from build123d import *

# Parameters (mm, degrees)
SKETCH_2_W                       = 40
SKETCH_2_H                       = 17
SM_BASE_FLANGE_1_DEPTH           = 2
SM_EDGE_FLANGE_1_STRIP_W         = 9.4732
SM_EDGE_FLANGE_1_STRIP_H         = 2
SM_EDGE_FLANGE_1_STRIP_CUT_DEPTH = 40
SM_EDGE_FLANGE_1_DEPTH           = 40
SKETCH_10_R                      = 3.3
CUT_EXTRUDE_1_DEPTH              = 10
FILLET_1_R                       = 6
FILLET_2_R                       = 2


# Sheet-metal steps are written as plain solids
with BuildPart() as part:
    # Sketch 2 → 基体-法兰1 (new body)
    with BuildSketch(Plane.XY):
        Rectangle(SKETCH_2_W, SKETCH_2_H)
    extrude(amount=-SM_BASE_FLANGE_1_DEPTH)

    # 边线-法兰1 strip (across the edge) → 边线-法兰1 strip cut (cut)
    with BuildSketch(Plane(origin=(-20, 8.5, -2), x_dir=(0, -1, 0), z_dir=(1, 0, 0))):
        with Locations((-2, -1)):
            Rectangle(SM_EDGE_FLANGE_1_STRIP_W, SM_EDGE_FLANGE_1_STRIP_H)
    extrude(amount=SM_EDGE_FLANGE_1_STRIP_CUT_DEPTH, mode=Mode.SUBTRACT)

    # 边线-法兰1 section (across the edge) → 边线-法兰1 (add)
    with BuildSketch(Plane(origin=(-20, 8.5, -2), x_dir=(0, -1, 0), z_dir=(1, 0, 0))):
        with BuildLine():
            Line((0, 0.7366), (0, 13))
            Line((0, 13), (2, 13))
            Line((2, 13), (2, 0.7366))
            ThreePointArc((2, 0.7366), (2.215745145, 0.215745145), (2.7366, 0))
            Line((2.7366, 0), (2.7366, -2))
            ThreePointArc((2.7366, -2), (0.801531583, -1.198468417), (0, 0.7366))
        make_face()
    extrude(amount=SM_EDGE_FLANGE_1_DEPTH)

    # 草图10 → 切除-拉伸1 (cut)
    with BuildSketch(Plane(origin=(0, 0, -2), x_dir=(-1, 0, 0), z_dir=(0, 0, -1))):
        with Locations((-12.5, -2.5)):
            Circle(SKETCH_10_R)
        with Locations((12.5, -2.5)):
            Circle(SKETCH_10_R)
    extrude(amount=-CUT_EXTRUDE_1_DEPTH, mode=Mode.SUBTRACT)

    # 圆角1
    fillet_1_edges = [part.edges().sort_by_distance(p)[0] for p in [
        (20, -8.5, -1),
        (-20, -8.5, -1),
    ]]
    fillet(fillet_1_edges, radius=FILLET_1_R)

    # 圆角2
    fillet_2_edges = [part.edges().sort_by_distance(p)[0] for p in [
        (-20, 7.5, -15),
        (20, 7.5, -15),
    ]]
    fillet(fillet_2_edges, radius=FILLET_2_R)


solid = part.part
CAD build for the part. Positions are in the model's coordinates, mm. A direction names the side the tool comes from. Coordinates: 2 decimals unless noted, no trailing zeros. Loops run counter-clockwise (first coordinate to the right, second up) from the corner with the lowest first, then second, coordinate; pieces in that order, holes last. Notation, with made-up numbers: (-2, 59.5) -> (25, 59.5) arc R22 cw to (25, 68.5) -> close; hole circle Ø9 at (4, 78.25). An arc over 180 degrees is marked (long way). One line per item, written item: value.
1. Flat gauge pin, fed straight in: P1, Ø7, axis at x = -3, y = 1.5, coming from the -Z side. Where does the tip first touch, or does it go through?
Answers:
P1: stops at z = -2
2. Slice it at D-D on y = 7.75. Write the cut outline in (x, z).
Answers:
outline: (-20, -13) arc R2 ccw to (-18, -15) -> (18, -15) arc R2 ccw to (20, -13) -> (20, -0.85) -> (-20, -0.85) -> close
3. Drill centre lines: line 1 (Y direction, x = -4.5, z = -12); line 2 (Z direction, x = 16, y = 4.25); line 3 (Y direction, x = -12.5, z = -1). Where is each one in solid material? Low to high. Write a range as [from, to].
Answers:
line 1: y = [6.5, 8.5]
line 2: z = [-2, 0]
line 3: y = [-8.5, -5.8], [0.8, 7.88]
4. Pull direction Y, two halves, no side cores. Call faces 1 (the face through (0, 8.5, -9)), 2 (the face through (-19.43, 7.49, -14.4)), 3 (the face through (-9.2, -2.4, -1)), 4 (the face through (18.289, -6.696, -1.014)): pulls with the +Y half, pulls with the -Y half, needs draft (parallel to the pull), parting line crosses it, or undercut.
Answers:
face 1: pulls with the +Y half
face 2: needs draft
face 3: undercut
face 4: pulls with the -Y half
5. Which spindle directions (+Z, -Z, +X, -X, +Y, -Y) get a long thin tool onto all of the face, cutting with end or side? Do faces 5 (the face through (0, 6.5, -9)), 6 (the face through (0, 8, -15)). Say none if no direction does.
Answers:
face 5: -Z, +X, -X, -Y
face 6: -Z, +X, -X, +Y, -Y
6. Slice it at B-B on z = -1.25. Write the cut outline in (x, y), and give its area (3 significant figures).
Answers:
outline: (-20, -2.5) arc R6 ccw to (-14, -8.5) -> (14, -8.5) arc R6 ccw to (20, -2.5) -> (20, 8.06) -> (-20, 8.06) -> close; hole circle Ø6.6 at (-12.5, -2.5); hole circle Ø6.6 at (12.5, -2.5)
area: 579 mm^2
7. Slice it at C-C on x = -5.5. Write the cut outline in (y, z), and give its area (3 significant figures).
Answers:
outline: (-8.5, -2) -> (5.76, -2) arc R0.74 cw to (6.5, -2.74) -> (6.5, -15) -> (8.5, -15) -> (8.5, -2.74) arc R2.74 ccw to (5.76, 0) -> (-8.5, 0) -> close
area: 58.5 mm^2
8. Slice it at A-A on x = -12.5. Write the cut outline in (y, z), and give its area (3 significant figures).
Answers:
outline: (-8.5, -2) -> (-5.8, -2) -> (-5.8, 0) -> (-8.5, 0) -> close; (0.8, -2) -> (5.76, -2) arc R0.74 cw to (6.5, -2.74) -> (6.5, -15) -> (8.5, -15) -> (8.5, -2.74) arc R2.74 ccw to (5.76, 0) -> (0.8, 0) -> close
area: 45.3 mm^2
